```python
from build123d import *


with BuildPart() as part:
    # Barrer1: sweep along a path in Croquis2
    with BuildLine(Plane.XY) as barrer1_path:
        Line((0, 172), (700, 172))
        ThreePointArc((700, 172), (872, 0), (700, -172))
        Line((700, -172), (0, -172))
        ThreePointArc((0, -172), (-172, 0), (0, 172))
    # Croquis3 → Barrer1 (sweep)
    with BuildSketch(Plane(origin=(0, 0, 0), x_dir=(0, 0, -1), z_dir=(1, 0, 0))):
        Polygon((-7, 172), (7, 172), (19.123999112, 198), (-19.123999112, 198), align=None)
    sweep(path=barrer1_path.line)


solid = part.part
```
CAD build for the part. Positions are in the model's coordinates, mm. A direction names the side the tool comes from. Round coordinates to 2 decimals unless told otherwise and drop trailing zeros. Write each loop counter-clockwise with the first axis right and the second up, starting at its lowest first coordinate (ties: lowest second). Pieces come first, ordered by that corner, then holes.
Item 1: Drill centre lines: L1, parallel to Y at x = 605, z = 4; L2, parallel to X at y = 8, z = -5; L3, parallel to X at y = 77, z = -11.5. Where is each one in solid material? Low to high.
Filled in:
L1: y = -198 to -172, 172 to 198
L2: x = -197.84 to -171.81, 871.81 to 897.84
L3: x = -182.41 to -164.52, 864.52 to 882.41
Item 2: Tool access for faces 1 (the flat face through (355, 198, 0)), 2 (the cylindrical face through (871.96, 3.78, -0.1)), 3 (the cylindrical face through (897.952, 4.354, 0.268)), 4 (the flat face through (354.9, 185.182, 13.147)), 5 (the conical face through (873.584, 3.818, -7.758)): list every direction of +Z, -Z, +X, -X, +Y, -Y with a clear straight run to the whole face (end or side of a thin tool).
Filled in:
face 1: +Z, -Z, +X, -X, +Y
face 2: +Z, -Z
face 3: +Z, -Z, +X
face 4: +Z
face 5: -Z
Item 3: Mould opens along Y. For faces 6 (the conical face through (-173.22, -3.81, 7.59)), 7 (the cylindrical face through (-197.952, -4.354, 0.268)), 8 (the cylindrical face through (-171.96, -3.78, -0.1)), 9 (the flat face through (345, -198, 0)) say: released by +Y, released by -Y, zero draft, split by the parting line, or undercut.
Filled in:
face 6: undercut
face 7: split by the parting line
face 8: undercut
face 9: released by -Y
Item 4: Band-saw the part on B-B on y = 0. Write the cut outline in (x, z).
Filled in:
outline: (-198, -19.12) - (-172, -7) - (-172, 7) - (-198, 19.12) - close; (872, -7) - (898, -19.12) - (898, 19.12) - (872, 7) - close
Item 5: Drop flat-ended pins along their axis: pin 1 Ø1.5 at (y, z) = (-139.5, -6) entering from -X; pin 2 Ø4 at (x, z) = (-19, 6.5) entering from -Y; pin 3 Ø2 at (y, z) = (-64, -5.5) entering from -X. Give the stop position or say it passes through.
Filled in:
pin 1: stops at x = -141.25
pin 2: stops at y = -197.27
pin 3: stops at x = -187.71
Item 6: Band-saw the part on A-A on x = 147.5. Write the cut outline in (y, z).
Filled in:
outline: (-198, -19.12) - (-172, -7) - (-172, 7) - (-198, 19.12) - close; (172, -7) - (198, -19.12) - (198, 19.12) - (172, 7) - close
